Verification items for the finished model (mm, model axes). Face numbers are marked on the shaded views. A direction names the side the tool comes from. Give positions to 0.01 mm unless a question says otherwise; leave off trailing zeros. Loops run counter-clockwise (first coordinate to the right, second up) from the corner with the lowest first, then second, coordinate; pieces in that order, holes last. Notation, with made-up numbers: M 53,81.5 L 107,81.5 A23 ccw 107,117.5 Z; hole C -8,-4.5 d5. An arc over 180 degrees is marked long. Use a Markdown table: item, result.
from build123d import *

# Parameters (mm, degrees)
SKETCH1_W           = 20
SKETCH1_H           = 10.66
BOSS_EXTRUDE1_DEPTH = 3.1
SKETCH2_R           = 1.27
CUT_EXTRUDE1_DEPTH  = 7.2
SKETCH3_W           = 0.5715
SKETCH3_H           = 3.3655
BOSS_EXTRUDE2_DEPTH = 3.6068
SKETCH4_W           = 1.778
SKETCH4_H           = 3.3
BOSS_EXTRUDE3_DEPTH = 1.3
CUT_EXTRUDE2_DEPTH  = 5.75


with BuildPart() as part:
    # Sketch1 → Boss-Extrude1 (new body, symmetric)
    with BuildSketch(Plane.XY):
        with Locations((0, 5.33)):
            Rectangle(SKETCH1_W, SKETCH1_H)
    extrude(amount=BOSS_EXTRUDE1_DEPTH, both=True)

    # Sketch2 → Cut-Extrude1 (cut, through all)
    with BuildSketch(Plane.XY.offset(3.1)):
        with Locations((4.699, 2.9337)):
            Circle(SKETCH2_R)
        with Locations((-4.699, 2.9337)):
            Circle(SKETCH2_R)
    extrude(amount=-CUT_EXTRUDE1_DEPTH, mode=Mode.SUBTRACT)

    # Sketch3 → Boss-Extrude2 (add)
    with BuildSketch(Plane.XZ):
        with Locations((-8.21425, 0)):
            Rectangle(SKETCH3_W, SKETCH3_H)
        Rectangle(SKETCH3_W, SKETCH3_H)
        with Locations((8.21425, 0)):
            Rectangle(SKETCH3_W, SKETCH3_H)
    extrude(amount=BOSS_EXTRUDE2_DEPTH)

    # Sketch4 → Boss-Extrude3 (add)
    with BuildSketch(Plane(origin=(0, 10.66, 0), x_dir=(1, 0, 0), z_dir=(0, 1, 0))):
        with Locations((2.761, 0)):
            Rectangle(SKETCH4_W, SKETCH4_H)
    extrude(amount=BOSS_EXTRUDE3_DEPTH)

    # Sketch5 → Cut-Extrude2 (cut, through all)
    with BuildSketch(Plane.XY.offset(1.65)):
        with BuildLine():
            Line((1.872, 11.96), (1.872, 11.71))
            ThreePointArc((1.872, 11.71), (2.29925846, 11.896310917), (2.761, 11.96))
            Line((2.761, 11.96), (1.872, 11.96))
        make_face()
        with BuildLine():
            ThreePointArc((2.761, 11.96), (3.22274154, 11.896310917), (3.65, 11.71))
            Line((3.65, 11.71), (3.65, 11.96))
            Line((3.65, 11.96), (2.761, 11.96))
        make_face()
    extrude(amount=-CUT_EXTRUDE2_DEPTH, mode=Mode.SUBTRACT)


solid = part.part
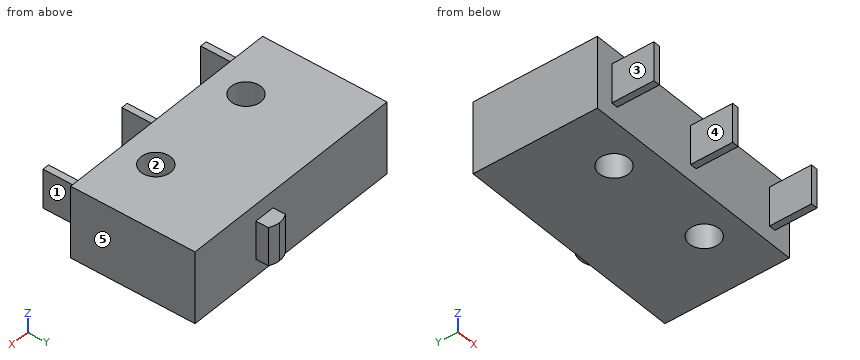
(1) Set-up check for the marked faces 3, 4 and 5: record each of +Z, -Z, +X, -X, +Y, -Y from which the full face is reachable in a straight line by a thin tool's end or side.
Results below:
| item | result |
|---|---|
| face 3 | +Z, -Z, -X, -Y |
| face 4 | +Z, -Z, -Y |
| face 5 | +Z, -Z, +X, +Y, -Y |
(2) Cross-section at A-A on y = -1.5. Record the cut outline in (x, z), then the cut area to 3 significant figures.
Results below:
| item | result |
|---|---|
| outline | M -8.5,-1.68 L -7.93,-1.68 L -7.93,1.68 L -8.5,1.68 Z; M -0.29,-1.68 L 0.29,-1.68 L 0.29,1.68 L -0.29,1.68 Z; M 7.93,-1.68 L 8.5,-1.68 L 8.5,1.68 L 7.93,1.68 Z |
| area | 5.77 mm^2 |
(3) Cross-section at C-C on z = -0.5. Record the cut outline in (x, y).
Results below:
| item | result |
|---|---|
| outline | M -10,0 L -8.5,0 L -8.5,-3.61 L -7.93,-3.61 L -7.93,0 L -0.29,0 L -0.29,-3.61 L 0.29,-3.61 L 0.29,0 L 7.93,0 L 7.93,-3.61 L 8.5,-3.61 L 8.5,0 L 10,0 L 10,10.66 L 3.65,10.66 L 3.65,11.71 A1.71 ccw 1.87,11.71 L 1.87,10.66 L -10,10.66 Z; hole C -4.7,2.93 d2.54; hole C 4.7,2.93 d2.54 |
(4) Gauge pin test, flat ends, axial feed: P1, Ø1.7, axis at y = -2, z = -0.5, coming from the +X side; P2, Ø1, axis at y = -1.5, z = 0, coming from the -X side; P3, Ø0.6, axis at x = -8, y = -2, coming from the +Z side; P4, Ø1.2, axis at y = 11, z = 1, coming from the -X side. Record the tip position at first contact, or that the pin passes through.
Results below:
| item | result |
|---|---|
| P1 | x = 8.5 |
| P2 | x = -8.5 |
| P3 | z = 1.68 |
| P4 | x = -10 |
(5) Material ranges on line 1 (X direction, y = 3, z = 1.5); line 2 (X direction, y = -1, z = 0.5); line 3 (Y direction, x = -5.5, z = 1), recorded low to high.
Results below:
| item | result |
|---|---|
| line 1 | -10 to -5.97, -3.43 to 3.43, 5.97 to 10 |
| line 2 | -8.5 to -7.93, -0.29 to 0.29, 7.93 to 8.5 |
| line 3 | 0 to 1.95, 3.92 to 10.66 |
(6) Draft check along Y on the marked faces 1 and 2. Enter one of: +Y half, -Y half, draft (parallel to the pull), parting line (faces both ways), or undercut.
Results below:
| item | result |
|---|---|
| face 1 | draft |
| face 2 | undercut |
(7) Cross-section at D-D on x = -8.25. Record the cut outline in (y, z).
Results below:
| item | result |
|---|---|
| outline | M -3.61,-1.68 L 0,-1.68 L 0,-3.1 L 10.66,-3.1 L 10.66,3.1 L 0,3.1 L 0,1.68 L -3.61,1.68 Z |
(8) Cross-section at B-B on x = -5.75. Record the cut outline in (y, z), then the cut area to 3 significant figures.
Results below:
| item | result |
|---|---|
| outline | M 0,-3.1 L 2.22,-3.1 L 2.22,3.1 L 0,3.1 Z; M 3.65,-3.1 L 10.66,-3.1 L 10.66,3.1 L 3.65,3.1 Z |
| area | 57.3 mm^2 |
